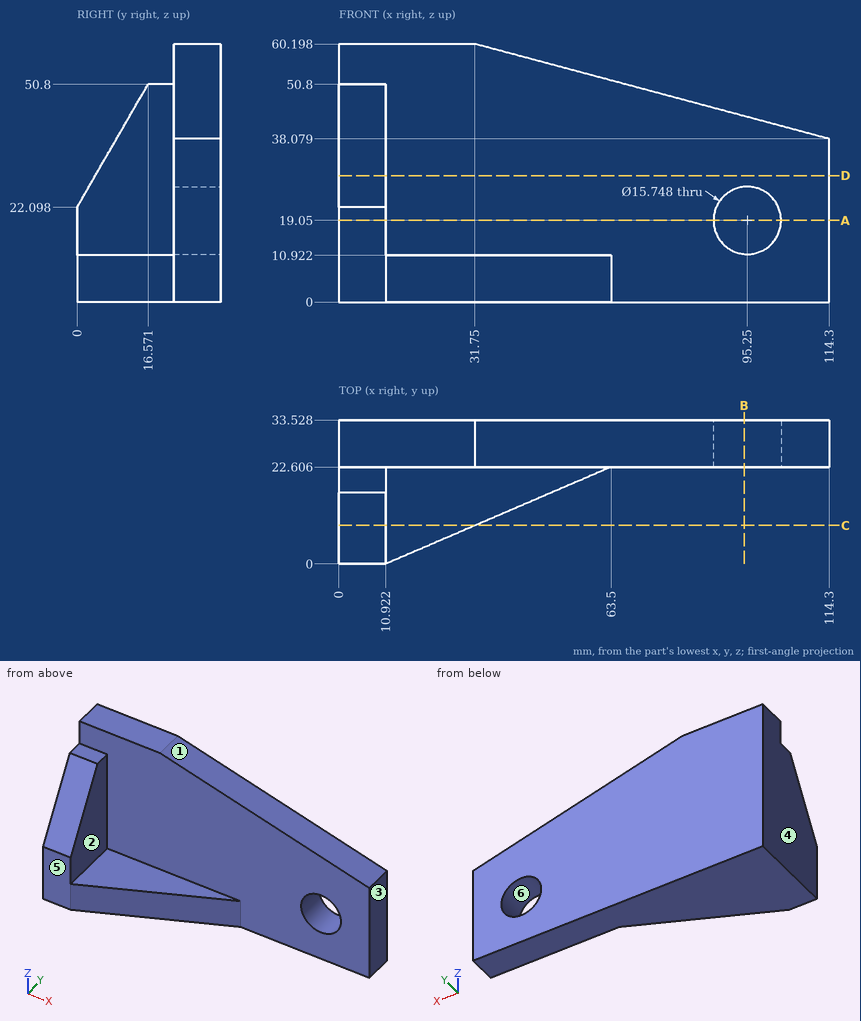
Here's the drawing with two shaded views (mm, measured from the low corner). I have some questions. A direction names the side the tool comes from. Coordinates: 2 decimals unless noted, no trailing zeros. Order: outer loops, then holes, each group sorted by start corner. A loop starts at its lowest first (then second) coordinate and runs counter-clockwise, first axis right, second up. Notation, with made-up numbers: (-22, 68.5) - (23, 68.5) arc R29 ccw to (23, 93.5) - close; hole circle Ø6 at (-9.75, -16). An arc over 180 degrees is marked (long way). Answer in a Markdown table with one row per item. Add a question column.
(1) If we section it at B-B, the plane x = 94.5: Please give me the cut outline in (y, z).
(2) If we section it at A-A, the plane z = 19.05: Please give me the cut outline in (x, y).
(3) On a 3-axis mill with a long thin cutter (end or side, diameter ignored), from which of +Z, -Z, +X, -X, +Y, -Y can I reach the whole of each face in a straight line? I mean the marked faces 1 and 2. Say none if no direction works.
(4) I need wall thicknesses on L1, parallel to X at y = 25, z = 19; L2, parallel to Z at x = 95, y = 25; L3, parallel to Y at x = 80, z = 46. Which ranges of each line are inside material? Lowest first, please.
(5) Will these pins go through, and if not, where does the flat tip stop? pin 1 (8 mm diameter, centred on x = 74, z = 53.5, fed in from +Y); pin 2 (4 mm diameter, centred on y = 17.5, z = 25.5, fed in from +X); pin 3 (5 mm diameter, centred on x = 6, y = 20.5, fed in from +Z); pin 4 (18 mm diameter, centred on x = 73.5, z = 38, fed in from -Y).
(6) If we section it at C-C, the plane y = 9: Please give me the cut outline in (x, z) (1 decimal), then the cut area to 3 significant figures.
(7) If we mould it in two halves opening along X, with no side actions, what happens to the marked faces 3, 4, 5 and 6? For each: released by +X, released by -X, zero draft, split by the parting line, or undercut.
(8) If we section it at D-D, the plane z = 29.5: Please give me the cut outline in (x, y), then the cut area to 3 significant figures.
Results are:
| question | item | result |
|---|---|---|
| 1 | outline | (22.61, 0) - (33.53, 0) - (33.53, 11.21) - (22.61, 11.21) - close; (22.61, 26.89) - (33.53, 26.89) - (33.53, 43.38) - (22.61, 43.38) - close |
| 2 | outline | (0, 0) - (10.92, 0) - (10.92, 22.61) - (87.38, 22.61) - (87.38, 33.53) - (0, 33.53) - close; (103.12, 22.61) - (114.3, 22.61) - (114.3, 33.53) - (103.12, 33.53) - close |
| 3 | face 1 | +Z, +X, +Y, -Y |
| 3 | face 2 | +Z, +X, -Y |
| 4 | L1 | x = 0 to 87.38, 103.12 to 114.3 |
| 4 | L2 | z = 0 to 11.18, 26.92 to 43.25 |
| 4 | L3 | y = 22.61 to 33.53 |
| 5 | pin 1 | passes through |
| 5 | pin 2 | stops at x = 10.92 |
| 5 | pin 3 | stops at z = 60.2 |
| 5 | pin 4 | stops at y = 22.61 |
| 6 | outline | (0, 0) - (31.9, 0) - (31.9, 10.9) - (10.9, 10.9) - (10.9, 37.7) - (0, 37.7) - close |
| 6 | area | 640 mm2 |
| 7 | face 3 | released by +X |
| 7 | face 4 | released by -X |
| 7 | face 5 | zero draft |
| 7 | face 6 | undercut |
| 8 | outline | (0, 4.27) - (10.92, 4.27) - (10.92, 22.61) - (114.3, 22.61) - (114.3, 33.53) - (0, 33.53) - close |
| 8 | area | 1,450 mm2 |
